from build123d import *

# Parameters (mm, degrees)
CUT_EXTRUDE_2_DEPTH      = 12
PATTERN_CIRCULAR_1_COUNT = 53
SKETCH_4_R               = 4
CUT_EXTRUDE_3_DEPTH      = 18


with BuildPart() as part:
    # 草图1 → 旋转1 (revolve)
    with BuildSketch(Plane.XY):
        Polygon((0, 17), (4, 17), (4, 14), (6.44, 14), (6.44, 11), (9.5, 11), (9.5, 3), (6.44, 3), (6.44, 0), (0, 0), align=None)
    revolve(axis=Axis((0, 17, 0), (0, -1, 0)))

    # 草图2 → 切除-拉伸2 (cut, through all)
    with BuildSketch(Plane(origin=(0, 11, 0), x_dir=(1, 0, 0), z_dir=(0, 1, 0))):
        with BuildLine():
            Line((0, 8), (1.396758286, 9.396758286))
            ThreePointArc((1.396758286, 9.396758286), (0, 9.5), (-1.396758286, 9.396758286))
            Line((-1.396758286, 9.396758286), (0, 8))
        make_face()
    cut_extrude_2 = extrude(amount=-CUT_EXTRUDE_2_DEPTH, mode=Mode.SUBTRACT)

    # 阵列(圆周)1: 切除-拉伸2 ×53 about axis
    pattern_circular_1_axis = Axis((0, 0, 0), (0, 1, 0))
    for i in range(1, PATTERN_CIRCULAR_1_COUNT):
        add(cut_extrude_2.rotate(pattern_circular_1_axis, i * 360 / PATTERN_CIRCULAR_1_COUNT), mode=Mode.SUBTRACT)

    # 草图4 → 切除-拉伸3 (cut, through all)
    with BuildSketch(Plane(origin=(0, 17, 0), x_dir=(1, 0, 0), z_dir=(0, 1, 0))):
        Circle(SKETCH_4_R)
    extrude(amount=-CUT_EXTRUDE_3_DEPTH, mode=Mode.SUBTRACT)


solid = part.part
Could you check a few things on this model? Use its own coordinates, in mm. A direction names the side the tool comes from. Coordinates: 2 decimals unless noted, no trailing zeros. Order: outer loops, then holes, each group sorted by start corner. A loop starts at its lowest first (then second) coordinate and runs counter-clockwise, first axis right, second up.
Q1. Suppose I cut it at D-D on z = 5.5. Please give me the cut outline in (x, y).
Q2. Suppose I cut it at A-A on z = 0. Please give me the cut outline in (x, y), and give its area (3 significant figures).
Q3. Please list where these lines run through material, in increasing order: L1, parallel to X at y = 8.5, z = 2.5; L2, parallel to X at y = 6.5, z = 0; L3, parallel to Y at x = -4.25, z = -5.75.
Q4. Suppose I cut it at B-B on y = 2.5. Please give me the cut outline in (x, z), and give its area (3 significant figures).
Q5. Which directions (+Z, -Z, +X, -X, +Y, -Y) give clear straight access to the entire face, cutting with the end or side of a thin tool? Please do faces 1 (the cylindrical face through (-1.396, 12.479, -6.287)), 2 (the flat face through (-6, 3, -3)), 3 (the flat face through (3, 0, 3)).
Q6. Suppose I cut it at C-C on x = -0.25. Please give me the cut outline in (y, z), and give its area (3 significant figures).
Q7. Will these pins go through, and if not, where does the flat tip stop? pin 1 (6.5 mm diameter, centred on x = 0, z = 0, fed in from -Y); pin 2 (2 mm diameter, centred on x = -0.5, y = 1.5, fed in from +Z).
Answer:
1. outline: (-6.26, 3) - (-3.35, 3) - (-3.35, 0) - (3.35, 0) - (3.35, 3) - (6.26, 3) - (6.26, 11) - (3.35, 11) - (3.35, 14) - (-3.35, 14) - (-3.35, 11) - (-6.26, 11) - close
2. outline: (-8.25, 3) - (-6.44, 3) - (-6.44, 0) - (-4, 0) - (-4, 14) - (-6.44, 14) - (-6.44, 11) - (-8.25, 11) - close; (4, 0) - (6.44, 0) - (6.44, 3) - (8.25, 3) - (8.25, 11) - (6.44, 11) - (6.44, 14) - (4, 14) - close
2. area: 97.2 mm2
3. L1: x = -7.7 to -3.12, 3.12 to 7.7
3. L2: x = -8.25 to -4, 4 to 8.25
3. L3: y = 3 to 11
4. outline: circle Ø12.88 at (0, 0); hole circle Ø8 at (0, 0)
4. area: 80.0 mm2
5. face 1: +Y
5. face 2: -Y
5. face 3: +Z, -Z, +X, -X, -Y
6. outline: (0, -6.44) - (3, -6.44) - (3, -8.25) - (11, -8.25) - (11, -6.44) - (14, -6.44) - (14, -3.99) - (0, -3.99) - close; (0, 3.99) - (14, 3.99) - (14, 6.44) - (11, 6.44) - (11, 8.24) - (3, 8.24) - (3, 6.44) - (0, 6.44) - close
6. area: 97.3 mm2
7. pin 1: passes through
7. pin 2: stops at z = 6.44
